Read the model definition and answer for the solid it produces. Units are mm, in the model's axes. A direction names the side the tool comes from. Round coordinates to 2 decimals unless told otherwise and drop trailing zeros. Order: outer loops, then holes, each group sorted by start corner. A loop starts at its lowest first (then second) coordinate and runs counter-clockwise, first axis right, second up. Notation, with made-up numbers: (69.25, 63.5) - (95.25, 63.5) arc R24 ccw to (95.25, 81.5) - close; hole circle Ø8 at (61, -30). An arc over 180 degrees is marked (long way). One line per question, with ' | ' between items. Start each with the question number.
1) For faces 1 (the cylindrical face through (2.465, 74.395, -78.276)), 2 (the flat face through (2, 93.548, -57)), 3 (the flat face through (2, 93, -64.795)), determine the directions among +Z, -Z, +X, -X, +Y, -Y from which every point of the face is accessible in a straight line to the end or side of a thin tool.
2) The part is cut by section A-A, the plane x = 4.15. Give the vertices of the cut face in (y, z).
3) The part is cut by section B-B, the plane z = -76. Give the vertices of the cut face in (x, y), plus the area to 3 significant figures.
4) The part is cut by section C-C, the plane y = 76.25. Give the vertices of the cut face in (x, z), plus the area to 3 significant figures.
5) The part is cut by section D-D, the plane z = -61.75. Give the vertices of the cut face in (x, y).
6) The mould has two halves that part along Z. Classify faces 4 (the flat face through (2, 69.944, -76)), 5 (the cylindrical face through (2.465, 85.609, -78.276)), 6 (the cylindrical face through (2.465, 83.843, -52.703)), 7 (the cylindrical face through (2.465, 71.085, -79.643)): pulls with the +Z half, pulls with the -Z half, needs draft (parallel to the pull), parting line crosses it, or undercut.
7) Flat-ended cylindrical pins translate along their axes: pin 1 (1 mm diameter, centred on x = 4, z = -69.5, fed in from +Y); pin 2 (2 mm diameter, centred on y = 92, z = -69, fed in from -X); pin 3 (2.5 mm diameter, centred on x = 2.5, z = -57.5, fed in from +Y); pin 4 (1.5 mm diameter, centred on x = 3.5, y = 95, fed in from +Z). Find the tip coordinate at first contact, or state that the pin passes through.
8) Straight lines are drawn through the part: line 1 (Y direction, x = 2, z = -76.75); line 2 (Y direction, x = 2.95, z = -76.25); line 3 (Z direction, x = 2.45, y = 95). For each, find the intervals that lie inside material, in ascending order. Write a range as from..to.
from build123d import *

# Parameters (mm, degrees)
SKETCH1_R           = 4
SKETCH1_R_2         = 1.5
BOSS_EXTRUDE1_DEPTH = 5


with BuildPart() as part:
    # Sketch1 → Boss-Extrude1 (new body)
    with BuildSketch(Plane(origin=(0, 0, 0), x_dir=(0, 0, -1), z_dir=(1, 0, 0))):
        with Locations((76.845680628, 73.944481469)):
            Circle(SKETCH1_R)
        with Locations((76.845680628, 73.944481469)):
            Circle(SKETCH1_R_2, mode=Mode.SUBTRACT)
        with Locations((76.845680628, 85.158009083)):
            Circle(SKETCH1_R)
        with Locations((76.845680628, 85.158009083)):
            Circle(SKETCH1_R_2, mode=Mode.SUBTRACT)
        with BuildLine():
            Line((80.845680628, 73.944481469), (80.845680628, 85.158009083))
            ThreePointArc((80.845680628, 85.158009083), (74.017253503, 82.329581958), (76.845680628, 89.158009083))
            Line((76.845680628, 89.158009083), (64.794938344, 89.158009083))
            Line((64.794938344, 89.158009083), (64.794938344, 96.547739715))
            Line((64.794938344, 96.547739715), (61.386991095, 96.547739715))
            Line((61.386991095, 96.547739715), (61.386991095, 93.547739715))
            Line((61.386991095, 93.547739715), (51.550416078, 93.547739715))
            Line((51.550416078, 93.547739715), (51.550416078, 88.503490644))
            ThreePointArc((51.550416078, 88.503490644), (52.73489617, 83.782621152), (56.007737829, 80.180106847))
            Line((56.007737829, 80.180106847), (68.86071523, 71.621097672))
            ThreePointArc((68.86071523, 71.621097672), (71.508038403, 70.372808732), (74.403393479, 69.944481469))
            Line((74.403393479, 69.944481469), (76.845680628, 69.944481469))
            ThreePointArc((76.845680628, 69.944481469), (74.017253503, 76.772908593), (80.845680628, 73.944481469))
        make_face()
    extrude(amount=BOSS_EXTRUDE1_DEPTH)


solid = part.part
Values:
1) face 1: +X, -X | face 2: +Z, +X, -X, +Y | face 3: -Z, +X, -X, +Y
2) outline: (69.94, -76.85) arc R4 ccw to (73.94, -80.85) - (85.16, -80.85) arc R4 ccw to (89.16, -76.85) - (89.16, -64.79) - (96.55, -64.79) - (96.55, -61.39) - (93.55, -61.39) - (93.55, -51.55) - (88.5, -51.55) arc R10 ccw to (80.18, -56.01) - (71.62, -68.86) arc R10 ccw to (69.94, -74.4) - close; hole circle Ø3 at (73.94, -76.85); hole circle Ø3 at (85.16, -76.85)
3) outline: (0, 69.94) - (5, 69.94) - (5, 72.71) - (0, 72.71) - close; (0, 75.18) - (5, 75.18) - (5, 83.92) - (0, 83.92) - close; (0, 86.4) - (5, 86.4) - (5, 89.16) - (0, 89.16) - close | area: 71.3 mm^2
4) outline: (0, -80.85) - (5, -80.85) - (5, -61.91) - (0, -61.91) - close | area: 94.7 mm^2
5) outline: (0, 76.36) - (5, 76.36) - (5, 96.55) - (0, 96.55) - close
6) face 4: needs draft | face 5: undercut | face 6: pulls with the +Z half | face 7: pulls with the -Z half
7) pin 1: stops at y = 89.16 | pin 2: passes through | pin 3: stops at y = 93.55 | pin 4: stops at z = -61.39
8) line 1: y = 69.94..72.45, 75.44..83.66, 86.65..89.16 | line 2: y = 69.94..72.57, 75.32..83.78, 86.53..89.16 | line 3: z = -64.79..-61.39
